```python
from build123d import *

# Parameters (mm, degrees)
BLANKSKE_W        = 150
BLANKSKE_H        = 22
BLANK_DEPTH       = 12
TOOTHCUTSIM_DEPTH = 153.078926877
TEETHCUTS_COUNT   = 25
TEETHCUTS_PITCH   = 6.2831853


with BuildPart() as part:
    # BlankSke → Blank (new body)
    with BuildSketch(Plane.XY):
        with Locations((75, 11)):
            Rectangle(BLANKSKE_W, BLANKSKE_H)
    extrude(amount=-BLANK_DEPTH)

    # TooCutSkeSim → ToothCutSim (cut, through all)
    with BuildSketch(Plane.XY):
        Polygon((0.861870739, 17.5), (-0.861870739, 17.5), (-2.508981637, 22.0254), (2.508981637, 22.0254), align=None)
    toothcutsim = extrude(amount=-TOOTHCUTSIM_DEPTH, mode=Mode.SUBTRACT)

    # TeethCuts: ToothCutSim ×25
    with Locations(*[(i * TEETHCUTS_PITCH, 0, 0) for i in range(1, TEETHCUTS_COUNT)]):
        add(toothcutsim, mode=Mode.SUBTRACT)


solid = part.part
```
Here's how the part is built. I have some questions about the finished solid (model axes, mm). Round coordinates to 2 decimals unless told otherwise and drop trailing zeros.
1. If I drill on probe 1 along Y at (x, z) = (50, -1.5), over which ranges is the centre line in solid material (lowest first)?
Answers:
probe 1: y = 0 to 17.5
2. Suppose I cut it at A-A, the plane y = 20.75. Give the number of separate pieces and of enclosed holes in the cut face, and give its area (3 significant figures).
Answers:
separate pieces: 24
enclosed holes: 0
area: 632 mm2
3. Will this pin go through, and if not, where does the flat tip stop? pin 1 (0.5 mm diameter, centred on x = 125.5, z = -7, fed in from +Y).
Answers:
pin 1: stops at y = 17.5
4. Thinking about a two-plate mould opening in X: for faces 1 (the face through (58.24, 19.78, -5.92)), 2 (the face through (74, 9, -12)), 3 (the face through (67.446, 19.718, -5.916)), which applies, released by +X, released by -X, zero draft, split by the parting line, or undercut?
Answers:
face 1: undercut
face 2: zero draft
face 3: undercut
